Read the model definition and answer for the solid it produces. Units are mm, in the model's axes. Face numbers are marked on the shaded views. A direction names the side the tool comes from. Round coordinates to 2 decimals unless told otherwise and drop trailing zeros. Order: outer loops, then holes, each group sorted by start corner. A loop starts at its lowest first (then second) coordinate and runs counter-clockwise, first axis right, second up. Notation, with made-up numbers: M -37.75,-4 L -2.75,-4 A20 ccw -2.75,14 Z; hole C 51.25,24.5 d2. An arc over 180 degrees is marked long. Answer as CSV lines item,"result".
```python
from build123d import *

# Parameters (mm, degrees)
F1_DEPTH = 10.16


with BuildPart() as f1:
    # F0 (on Right) → F1 (new body)
    with BuildSketch(Plane.YZ):
        with BuildLine():
            Line((0, -3.692769), (0, 34.465846))
            Line((0, 34.465846), (-8.308733, 34.465846))
            Line((-8.308733, 34.465846), (-8.308733, -3.692769))
            ThreePointArc((-8.308733, -3.692769), (-21.848886, -17.232923), (-35.38904, -3.692769))
            Line((-35.38904, -3.692769), (-43.390039, -3.692769))
            ThreePointArc((-43.390039, -3.692769), (-21.69502, -25.387789), (0, -3.692769))
        make_face()
    extrude(amount=F1_DEPTH)


solid = f1.part
```
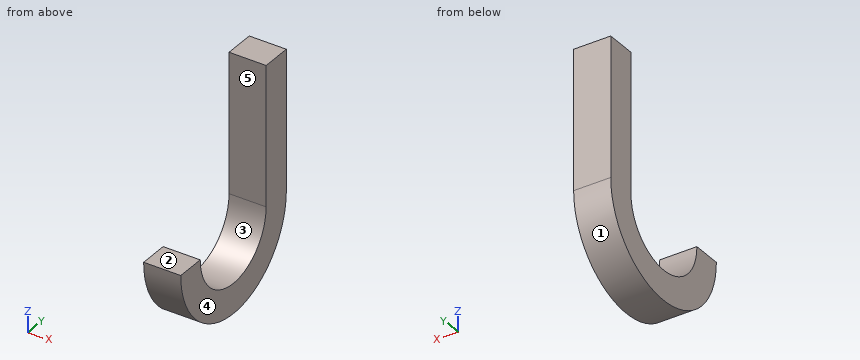
Item 1: A cutting plane is placed at D-D, the plane y = -9.5. Determine the outline of the cut face in (x, z).
Ans:
outline,"M 0,-21.64 L 10.16,-21.64 L 10.16,-9.25 L 0,-9.25 Z"
Item 2: Find the intervals of material crossed by probe 1 along Z at (x, y) = (7, -21.5); probe 2 along Y at (x, z) = (4.25, 11.5); probe 3 along Y at (x, z) = (1, -15), in increasing order. Write a range as [from, to].
Ans:
probe 1,"[-25.39, -17.23]"
probe 2,"[-8.31, 0]"
probe 3,"[-40.21, -29.3], [-14.4, -3.18]"
Item 3: A cutting plane is placed at A-A, the plane z = -4.5. Determine the outline of the cut face in (x, y).
Ans:
outline,"M 0,-43.38 L 10.16,-43.38 L 10.16,-35.36 L 0,-35.36 Z; M 0,-8.33 L 10.16,-8.33 L 10.16,-0.02 L 0,-0.02 Z"
Item 4: Determine the mould class of the marked faces 1, 2 and 3 for opening direction Y: +Y half, -Y half, draft (parallel to the pull), parting line (faces both ways), or undercut.
Ans:
face 1,"parting line"
face 2,"draft"
face 3,"undercut"
Item 5: Flat-ended cylindrical pins translate along their axes: pin 1 (5 mm diameter, centred on x = 2, z = 11, fed in from -Y); pin 2 (4 mm diameter, centred on x = 1.5, y = -11.5, fed in from -Z); pin 3 (3 mm diameter, centred on x = 3.5, y = -8.5, fed in from -Z). Find the tip coordinate at first contact, or state that the pin passes through.
Ans:
pin 1,"y = -8.31"
pin 2,"z = -23.78"
pin 3,"z = -21.97"
Item 6: A cutting plane is placed at C-C, the plane z = 30. Determine the outline of the cut face in (x, y), and give its area (3 significant figures).
Ans:
outline,"M 0,-8.31 L 10.16,-8.31 L 10.16,0 L 0,0 Z"
area,"84.4 mm2"
Item 7: A tool of negligible diameter and unlimited length cuts with its end or side. For the marked faces 4 and 5, from which of +Z, -Z, +X, -X, +Y, -Y can it reach the whole face along a straight path? Write none if from no direction.
Ans:
face 4,"+Z, -Z, +X, +Y, -Y"
face 5,"+Z, +X, -X, -Y"
